Work out the finished part from the listing and answer in its coordinate system (mm). A direction names the side the tool comes from. Coordinates: 2 decimals unless noted, no trailing zeros. Write each loop counter-clockwise with the first axis right and the second up, starting at its lowest first coordinate (ties: lowest second). Pieces come first, ordered by that corner, then holes. Notation, with made-up numbers: (38, 47) -> (71, 47) arc R18 cw to (71, 62) -> close; hole circle Ø11 at (88.5, -8). An arc over 180 degrees is marked (long way). Write each question's results on one line, items separated by ' | '. Start each with the question number.
from build123d import *

# Parameters (mm, degrees)
BOSS_EXTRUDE1_DEPTH     = 190.5
F_6_CLEARANCE_HOLE1_D   = 3.7973
CUT_EXTRUDE1_DEPTH      = 32.75
SKETCH6_W               = 25.4
SKETCH6_H               = 15.24
CUT_EXTRUDE2_DEPTH      = 191.5
CUT_EXTRUDE2_DEPTH_BACK = 191.5
F_6_CLEARANCE_HOLE2_D   = 3.7973


with BuildPart() as part:
    # Sketch1 → Boss-Extrude1 (new body, symmetric)
    with BuildSketch(Plane(origin=(0, 0, 0), x_dir=(0, 0, -1), z_dir=(1, 0, 0))):
        Polygon((0, 0), (31.75, 0), (31.75, 3.048), (3.048, 3.048), (3.048, 31.75), (0, 31.75), align=None)
    extrude(amount=BOSS_EXTRUDE1_DEPTH, both=True)

    # #6 Clearance Hole1 (through all)
    with Locations(Plane.XY):
        with Locations((135.9, 27), (135.9, 11), (99.5, 27), (99.468, 11), (-121.868, 27), (-121.868, 11), (-85.468, 11), (-85.468, 27)):
            Hole(F_6_CLEARANCE_HOLE1_D / 2)

    # Sketch5 → Cut-Extrude1 (cut, through all)
    with BuildSketch(Plane.XY):
        with BuildLine():
            Line((149.877, 41.148), (149.877, 19.558))
            ThreePointArc((149.877, 19.558), (150.992923164, 16.863923164), (153.687, 15.748))
            Line((153.687, 15.748), (186.69, 15.748))
            ThreePointArc((186.69, 15.748), (189.384076836, 14.632076836), (190.5, 11.938))
            Line((190.5, 11.938), (190.5, -9.652))
            Line((190.5, -9.652), (198.12, -9.652))
            Line((198.12, -9.652), (198.12, 41.148))
            Line((198.12, 41.148), (149.877, 41.148))
        make_face()
        with BuildLine():
            Line((-198.12, 41.148), (-149.877, 41.148))
            Line((-149.877, 41.148), (-149.877, 19.558))
            ThreePointArc((-149.877, 19.558), (-150.992923164, 16.863923164), (-153.687, 15.748))
            Line((-153.687, 15.748), (-186.69, 15.748))
            ThreePointArc((-186.69, 15.748), (-189.384076836, 14.632076836), (-190.5, 11.938))
            Line((-190.5, 11.938), (-190.5, -9.652))
            Line((-190.5, -9.652), (-198.12, -9.652))
            Line((-198.12, -9.652), (-198.12, 41.148))
        make_face()
    extrude(amount=-CUT_EXTRUDE1_DEPTH, mode=Mode.SUBTRACT)

    # Sketch6 → Cut-Extrude2 (cut, two sides)
    with BuildSketch(Plane(origin=(0, 0, 0), x_dir=(0, 0, -1), z_dir=(1, 0, 0))) as cut_extrude2_sk:
        with Locations((20.32, 0)):
            Rectangle(SKETCH6_W, SKETCH6_H)
    extrude(amount=CUT_EXTRUDE2_DEPTH, mode=Mode.SUBTRACT)
    extrude(cut_extrude2_sk.sketch, amount=-CUT_EXTRUDE2_DEPTH_BACK, mode=Mode.SUBTRACT)

    # #6 Clearance Hole2 (through all)
    with Locations(Plane.XY):
        with Locations((-63.448, 27), (-63.448, 11)):
            Hole(F_6_CLEARANCE_HOLE2_D / 2)


solid = part.part
1. Find the intervals of material crossed by L1, parallel to Y at x = -63, z = -1.5; L2, parallel to Z at x = 108, y = 24; L3, parallel to X at y = 20, z = -2.5, in increasing order.
2. For faces 1 (the face through (3, 0, -4)), 2 (the face through (3, 17, -3.048)), determine the directions among +Z, -Z, +X, -X, +Y, -Y from which every point of the face is accessible in a straight line to the end or side of a thin tool.
3. Find section B-B on x = -7.5. Give the vertices of the cut face in (y, z).
4. Find section A-A on z = -1.5. Give the number of separate pieces and of enclosed holes in the cut face, and give its area (3 significant figures).
5. Given pin 1 Ø2.5 at (y, z) = (27.5, -1.5) entering from -X; pin 2 Ø12 at (x, y) = (95, 17) entering from -Z; pin 3 Ø2.5 at (x, z) = (164, -2) entering from +Y, each flat-ended and moving along its own axis, determine where each tip first touches the part or whether it passes through.
Ans:
1) L1: y = 0 to 9.15, 12.85 to 25.15, 28.85 to 31.75 | L2: z = -3.05 to 0 | L3: x = -149.88 to 149.88
2) face 1: +Z, -Z, +X, -X, -Y | face 2: -Z, +X, -X, +Y
3) outline: (0, -7.62) -> (3.05, -7.62) -> (3.05, -3.05) -> (31.75, -3.05) -> (31.75, 0) -> (0, 0) -> close
4) separate pieces: 1 | enclosed holes: 10 | area: 10,700 mm²
5) pin 1: stops at x = -149.88 | pin 2: stops at z = -3.05 | pin 3: stops at y = 15.75
